from build123d import *

# Parameters (mm, degrees)
F1_DEPTH  = 15
F3_DEPTH  = 2
F4_R      = 1.5
F5_DEPTH  = 25
F7_DEPTH  = 4
F8_SIZE   = 3
F10_DEPTH = 3.5
F11_DEPTH = 1


with BuildPart() as f1:
    # F0 (on Front) → F1 (new body)
    with BuildSketch(Plane.XZ):
        Polygon((-28.5, 38), (0, 38), (28.5, 38), (28.5, 0), (37.7, 0), (37.7, 1.5), (29.7, 1.5), (29.7, 39.5), (0, 39.5), (-29.7, 39.5), (-29.7, 1.5), (-37.7, 1.5), (-37.7, 0), (-28.5, 0), align=None)
    extrude(amount=F1_DEPTH)

    # F2 (on face) → F3 (join)
    with BuildSketch(Plane(origin=(0, 0, 0), x_dir=(-1, 0, 0), z_dir=(0, 1, 0))):
        Polygon((-28.5, 11), (-28.5, 8), (-2, 8), (2, 8), (28.5, 8), (28.5, 11), (2, 11), (2, 25), (28.5, 25), (28.5, 28), (2, 28), (2, 38), (-2, 38), (-2, 28), (-28.5, 28), (-28.5, 25), (-2, 25), (-2, 11), align=None)
    extrude(amount=-F3_DEPTH)

    # F4 (on face) → F5 (cut)
    with BuildSketch(Plane.XY.offset(1.5)):
        with Locations((-33.7, -7.5)):
            Circle(F4_R)
        with Locations((33.7, -7.5)):
            Circle(F4_R)
    extrude(amount=-F5_DEPTH, mode=Mode.SUBTRACT)

    # F6 (on Right) → F7 (join, symmetric)
    with BuildSketch(Plane.YZ):
        Polygon((-12.2525225805, 39.5), (-15, 40.5), (-23, 40.5), (-23, 38), (-23, 36.5), (-21.5, 36.5), (-20, 38), (-15, 38), (-15, 39.5), align=None)
    extrude(amount=F7_DEPTH, both=True)

    # F8
    f8_edges = [f1.edges().sort_by_distance(p)[0] for p in [
        (4, -15, 38.75),
        (-4, -15, 38.75),
    ]]
    chamfer(f8_edges, length=F8_SIZE)

    # F9 (on face) → F10 (join)
    with BuildSketch(Plane(origin=(0, 0, 0), x_dir=(-1, 0, 0), z_dir=(0, 1, 0))):
        Polygon((-29.7, 1.5), (-29.7, 16.5), (-31.7, 16.5), (-37.7, 3.5), (-37.7, 1.5), align=None)
        Polygon((29.7, 1.5), (37.7, 1.5), (37.7, 3.5), (31.7, 16.5), (29.7, 16.5), align=None)
    extrude(amount=-F10_DEPTH)

    # F11 (add): faces of the model
    f11_faces = [f1.faces().sort_by_distance(p)[0] for p in [
        (-37.5240340942, -7.5, 0),
        (28.6759659058, -7.5, 0),
    ]]
    extrude(f11_faces, amount=F11_DEPTH)


solid = f1.part
CAD build for the part. Positions are in the model's coordinates, mm. A direction names the side the tool comes from. Round coordinates to 2 decimals unless told otherwise and drop trailing zeros. Write each loop counter-clockwise with the first axis right and the second up, starting at its lowest first coordinate (ties: lowest second). Pieces come first, ordered by that corner, then holes. Notation, with made-up numbers: (-31.5, 19.5) -> (-6.5, 19.5) arc R17 ccw to (-6.5, 24.5) -> close; hole circle Ø5 at (7.25, 22). An arc over 180 degrees is marked (long way). Answer as a JSON object with one key per item and string values.
(1) Band-saw the part on C-C, the plane z = 17.5. List the corners of the cut face in (x, y).
Reported:
{"outline": "(-29.7, -15) -> (-28.5, -15) -> (-28.5, 0) -> (-29.7, 0) -> close; (-2, -2) -> (2, -2) -> (2, 0) -> (-2, 0) -> close; (28.5, -15) -> (29.7, -15) -> (29.7, 0) -> (28.5, 0) -> close"}
(2) Band-saw the part on D-D, the plane x = -33.7. List the corners of the cut face in (y, z).
Reported:
{"outline": "(-15, -1) -> (-9, -1) -> (-9, 1.5) -> (-15, 1.5) -> close; (-6, -1) -> (0, -1) -> (0, 12.17) -> (-3.5, 12.17) -> (-3.5, 1.5) -> (-6, 1.5) -> close"}
(3) Which spindle directions (+Z, -Z, +X, -X, +Y, -Y) get a long thin tool onto all of the face, cutting with end or side? Do faces 4 (the face through (29, -15, 21)), 5 (the face through (15, -1, 11)), 6 (the face through (-4, -20, 39)), 7 (the face through (4, -20, 39)), 8 (the face through (-31, -2, 16.5)). Say none if no direction does.
Reported:
{"face 4": "+Z, -Z, +X, -Y", "face 5": "+Y, -Y", "face 6": "+Z, -X, -Y", "face 7": "+Z, +X, -Y", "face 8": "+Z, -X, +Y, -Y"}
(4) Two-plate mould, pull along X, no slides. Class faces 1 (the face through (-5, -17, 39)), 2 (the face through (0, -8, 38)), 3 (the face through (-33, -3.5, 7)): +X half, -X half, draft (parallel to the pull), parting line (faces both ways), or undercut.
Reported:
{"face 1": "-X half", "face 2": "undercut", "face 3": "draft"}
(5) Band-saw the part on B-B, the plane y = -7.5. List the corners of the cut face in (x, z).
Reported:
{"outline": "(-37.7, -1) -> (-35.2, -1) -> (-35.2, 1.5) -> (-37.7, 1.5) -> close; (-32.2, -1) -> (-28.5, -1) -> (-28.5, 38) -> (28.5, 38) -> (28.5, -1) -> (32.2, -1) -> (32.2, 1.5) -> (29.7, 1.5) -> (29.7, 39.5) -> (-29.7, 39.5) -> (-29.7, 1.5) -> (-32.2, 1.5) -> close; (35.2, -1) -> (37.7, -1) -> (37.7, 1.5) -> (35.2, 1.5) -> close"}
(6) Probe probe 1 along X at (y, z) = (-1.5, 20.5); probe 2 along Z at (x, y) = (26.5, -1.75); probe 3 along Y at (x, z) = (33.7, 0.45). List the from-to ranges inside material, lowest first. Write a range as [from, to].
Reported:
{"probe 1": "x = [-29.7, -28.5], [-2, 2], [28.5, 29.7]", "probe 2": "z = [8, 11], [25, 28], [38, 39.5]", "probe 3": "y = [-15, -9], [-6, 0]"}
(7) Pin check, flat tips, straight feed: P1, Ø1.5, axis at y = -2.5, z = 30.5, coming from the +X side; P2, Ø6, axis at x = 15.5, y = -3, coming from the +Z side; P3, Ø4, axis at x = 33.5, z = 10, coming from the -Y side; P4, Ø6, axis at y = -15.5, z = 3.5, coming from the +X side. Stop position of each tip, or through.
Reported:
{"P1": "stops at x = 29.7", "P2": "stops at z = 39.5", "P3": "stops at y = -3.5", "P4": "stops at x = 37.7"}
(8) Band-saw the part on A-A, the plane x = 15. List the corners of the cut face in (y, z), then the cut area to 3 significant figures.
Reported:
{"outline": "(-15, 38) -> (0, 38) -> (0, 39.5) -> (-15, 39.5) -> close; (-2, 8) -> (0, 8) -> (0, 11) -> (-2, 11) -> close; (-2, 25) -> (0, 25) -> (0, 28) -> (-2, 28) -> close", "area": "34.5 mm^2"}
